Here's the drawing with two shaded views (mm, measured from the low corner). I have some questions. Round coordinates to 2 decimals unless told otherwise and drop trailing zeros. Loops run counter-clockwise (first coordinate to the right, second up) from the corner with the lowest first, then second, coordinate; pieces in that order, holes last. Notation, with made-up numbers: (82, -5) -> (107, -5) arc R31 cw to (107, 26) -> close; hole circle Ø9 at (-5, -3.5). An arc over 180 degrees is marked (long way). Write item = value, one per line.
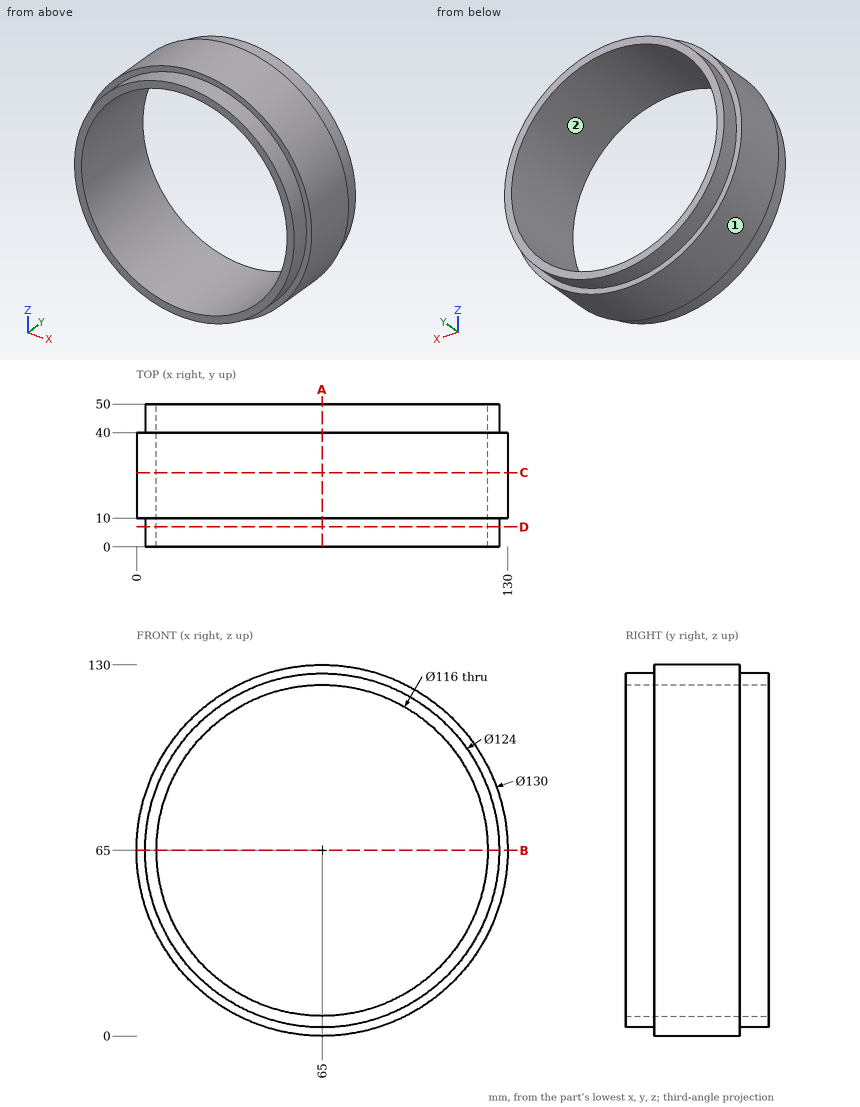
1. Suppose I cut it at A-A, the plane x = 65. List the corners of the cut face in (y, z) for me.
Entries:
outline = (0, 3) -> (10, 3) -> (10, 0) -> (40, 0) -> (40, 3) -> (50, 3) -> (50, 7) -> (0, 7) -> close; (0, 123) -> (50, 123) -> (50, 127) -> (40, 127) -> (40, 130) -> (10, 130) -> (10, 127) -> (0, 127) -> close
2. Suppose I cut it at D-D, the plane y = 7. List the corners of the cut face in (x, z) for me.
Entries:
outline = circle Ø124 at (65, 65); hole circle Ø116 at (65, 65)
3. I need wall thicknesses on line 1 (X direction, y = 16, z = 65); line 2 (Z direction, x = 66, y = 14); line 3 (Z direction, x = 108.5, y = 15). Which ranges of each line are inside material? Lowest first, please. Write a range as [from, to].
Entries:
line_1 = [0, 7], [123, 130]
line_2 = [0.01, 7.01], [122.99, 129.99]
line_3 = [16.7, 26.64], [103.36, 113.3]
4. I'm going to push flat-ended pins straight in: pin 1 (6 mm diameter, centred on x = 83, y = 26, fed in from -Z); pin 2 (8 mm diameter, centred on y = 27, z = 73.5, fed in from +X); pin 3 (3 mm diameter, centred on y = 24, z = 68.5, fed in from +X). Where does each tip first touch, or does it pass through?
Entries:
pin_1 = 1.75
pin_2 = 129.84
pin_3 = 129.97
5. We'd pull the mould along X, two halves only. Please class the marked faces 1 and 2: released by +X, released by -X, zero draft, split by the parting line, or undercut.
Entries:
face_1 = split by the parting line
face_2 = undercut
6. Suppose I cut it at C-C, the plane y = 26. List the corners of the cut face in (x, z) for me, and give its area (3 significant figures).
Entries:
outline = circle Ø130 at (65, 65); hole circle Ø116 at (65, 65)
area = 2,700 mm²
7. Suppose I cut it at B-B, the plane z = 65. List the corners of the cut face in (x, y) for me, and give its area (3 significant figures).
Entries:
outline = (0, 10) -> (3, 10) -> (3, 0) -> (7, 0) -> (7, 50) -> (3, 50) -> (3, 40) -> (0, 40) -> close; (123, 0) -> (127, 0) -> (127, 10) -> (130, 10) -> (130, 40) -> (127, 40) -> (127, 50) -> (123, 50) -> close
area = 580 mm²
